The listing builds one solid part. Answer for the finished solid, in the listing's coordinates (mm). A direction names the side the tool comes from. Give positions to 0.01 mm unless a question says otherwise; leave off trailing zeros. Order: outer loops, then holes, each group sorted by start corner. A loop starts at its lowest first (then second) coordinate and runs counter-clockwise, first axis right, second up. Notation, with made-up numbers: (-5.5, -17) - (39.5, -17) arc R32 ccw to (39.5, 18) - close; hole circle Ø4 at (39, 13). An arc over 180 degrees is marked (long way). Use CSV: the item, a comma, the result in double quotes.
```python
from build123d import *

# Parameters (mm, degrees)
F1_DEPTH = 35
F0_W     = 40
F0_H     = 30
F2_DEPTH = 25
F4_DEPTH = 30.001
F5_W     = 10
F5_H     = 20
F6_DEPTH = 80.001
F7_W     = 10
F7_H     = 10
F8_DEPTH = 80.001


with BuildPart() as f1:
    # F0 (on Front) → F1 (new body, symmetric)
    with BuildSketch(Plane.XZ):
        Polygon((0, 30), (0, 0), (110, 0), (110, 10), (80, 30), (70, 30), (30, 30), align=None)
    extrude(amount=F1_DEPTH, both=True)

    # F0 (on Front) → F2 (join, symmetric)
    with BuildSketch(Plane.XZ):
        with Locations((50, 45)):
            Rectangle(F0_W, F0_H)
    extrude(amount=F2_DEPTH, both=True)

    # F3 (on face) → F4 (cut, through all)
    with BuildSketch(Plane.XY.offset(30)):
        Polygon((0, -35), (30, -35), (0, -15), align=None)
        Polygon((0, 15), (30, 35), (0, 35), align=None)
    extrude(amount=-F4_DEPTH, mode=Mode.SUBTRACT)

    # F5 (on face) → F6 (cut, through all)
    with BuildSketch(Plane(origin=(30, 0, 0), x_dir=(0, -1, 0), z_dir=(-1, 0, 0))):
        with Locations((-20, 50)):
            Rectangle(F5_W, F5_H)
        with Locations((20, 50)):
            Rectangle(F5_W, F5_H)
    extrude(amount=-F6_DEPTH, mode=Mode.SUBTRACT)

    # F7 (on face) → F8 (cut, through all)
    with BuildSketch(Plane(origin=(30, 0, 0), x_dir=(0, -1, 0), z_dir=(-1, 0, 0))):
        with Locations((0, 55)):
            Rectangle(F7_W, F7_H)
    extrude(amount=-F8_DEPTH, mode=Mode.SUBTRACT)


solid = f1.part
```
Item 1: Which of the six approach directions +Z, -Z, +X, -X, +Y, -Y give full straight-line access (tool end or side, diameter ignored) to faces 1 (the face through (50, 5, 55)), 2 (the face through (50, -25, 35)), 3 (the face through (50, 20, 40)), 4 (the face through (70, 0, 41))?
Taken from the geometry:
face 1,"+Z, +X, -X"
face 2,"+Z, +X, -X, -Y"
face 3,"+Z, +X, -X, +Y"
face 4,"+Z, +X, +Y, -Y"
Item 2: The part is cut by section C-C (z = 4). Give the vertices of the cut face in (x, y), and give its area (3 significant figures).
Taken from the geometry:
outline,"(0, -15) - (30, -35) - (110, -35) - (110, 35) - (30, 35) - (0, 15) - close"
area,"7,100 mm^2"
Item 3: The part is cut by section A-A (y = -12). Give the vertices of the cut face in (x, z), and give its area (3 significant figures).
Taken from the geometry:
outline,"(0, 0) - (110, 0) - (110, 10) - (80, 30) - (70, 30) - (70, 60) - (30, 60) - (30, 30) - (0, 30) - close"
area,"4,200 mm^2"
Item 4: The mould has two halves that part along Y. Classify faces 5 (the face through (50, -10, 60)), 6 (the face through (50, -5, 55)), 7 (the face through (50, 15, 50)): +Y half, -Y half, draft (parallel to the pull), parting line (faces both ways), or undercut.
Taken from the geometry:
face 5,"draft"
face 6,"undercut"
face 7,"+Y half"
Item 5: Find the intervals of material crossed by line 1 along Z through (x, y) = (63.5, 19.5); line 2 along Z through (x, y) = (19.5, -22.5); line 3 along Y through (x, z) = (67, 36), in increasing order.
Taken from the geometry:
line 1,"0 to 40"
line 2,"0 to 30"
line 3,"-25 to 25"
Item 6: Each of these flat-tipped pins is pushed along its axis until it touches: pin 1 (3 mm diameter, centred on x = 51, y = -21.5, fed in from +Z); pin 2 (5 mm diameter, centred on y = 5, z = 37.5, fed in from +X); pin 3 (10 mm diameter, centred on x = 53.5, z = 47, fed in from -Y). Where does it stop, or does it pass through?
Taken from the geometry:
pin 1,"z = 40"
pin 2,"x = 70"
pin 3,"y = -15"
Item 7: The part is cut by section B-B (x = 51). Give the vertices of the cut face in (y, z), and give its area (3 significant figures).
Taken from the geometry:
outline,"(-35, 0) - (35, 0) - (35, 30) - (25, 30) - (25, 40) - (15, 40) - (15, 60) - (5, 60) - (5, 50) - (-5, 50) - (-5, 60) - (-15, 60) - (-15, 40) - (-25, 40) - (-25, 30) - (-35, 30) - close"
area,"3,100 mm^2"
Item 8: The part is cut by section D-D (z = 13.5). Give the vertices of the cut face in (x, y).
Taken from the geometry:
outline,"(0, -15) - (30, -35) - (104.75, -35) - (104.75, 35) - (30, 35) - (0, 15) - close"
